Check sheet for the modelled part. Datum: model origin and axes. Units: mm. A direction names the side the tool comes from. Give positions to 0.01 mm unless a question says otherwise; leave off trailing zeros. Order: outer loops, then holes, each group sorted by start corner. A loop starts at its lowest first (then second) coordinate and runs counter-clockwise, first axis right, second up. Notation, with made-up numbers: (-17, -20) -> (30, -20) arc R30 cw to (30, 2) -> close; hole circle Ø2 at (62, 3). An arc over 180 degrees is marked (long way). Answer in a Markdown table with one row per item. Add a question column.
(1) Cross-section at D-D (x = 3.25). Record the cut outline in (y, z), then the cut area to 3 significant figures.
(2) Set-up check for faces 4 (the face through (1.5, 0, 1)), 5 (the face through (0, -2, 3)): record each of +Z, -Z, +X, -X, +Y, -Y from which the full face is reachable in a straight line by a thin tool's end or side.
(3) Go/stop test with a flat-tipped pin: pin 1 (1.5 mm diameter, centred on x = 3.5, z = 2, fed in from -Y). Record where the tip stops, or that it passes through.
(4) Cross-section at C-C (z = 0.7). Record the cut outline in (x, y), then the cut area to 3 significant figures.
(5) Cross-section at A-A (y = 0). Record the cut outline in (x, z), then the cut area to 3 significant figures.
(6) Release check for a two-part mould opening along X. For faces 1 (the face through (0, -2, 0)), 2 (the face through (-1.5, 0, 1)), 3 (the face through (-0.59, -4.46, 1.48)) record: released by +X, released by -X, zero draft, split by the parting line, or undercut.
(7) Thickness scan on L1, parallel to Y at x = -0.75, z = 1.6; L2, parallel to Y at x = 0.5, z = 0.65; L3, parallel to X at y = 1, z = 0.75. Record the ranges inside material, lowest first. Write a range as [from, to].
Autodesk Inventor part; units mm, degrees
ref_plane "YZ Plane" through (0, 0, 0) normal (1, 0, 0) x (0, 1, 0)
ref_plane "XZ Plane" through (0, 0, 0) normal (0, 1, 0) x (-1, 0, 0)
ref_plane "XY Plane" through (0, 0, 0) normal (0, 0, 1) x (1, 0, 0)
sketch "Esboço1" plane through (0, 0, 0) normal (0, 0, 1) x (1, 0, 0)
  circle A0 centre (0, 0) radius 4.5
  line L0 (-1.5, 1.5) -> (1.5, 1.5)
  line L1 (1.5, 1.5) -> (1.5, -1.5)
  line L2 (1.5, -1.5) -> (-1.5, -1.5)
  line L3 (-1.5, -1.5) -> (-1.5, 1.5)
extrude "Extrusão1" add sketch "Esboço1" along normal blind 3
properties part number "TRAVA_HELICE"
Answer below:
| question | item | result |
|---|---|---|
| 1 | outline | (-3.11, 0) -> (3.11, 0) -> (3.11, 3) -> (-3.11, 3) -> close |
| 1 | area | 18.7 mm² |
| 2 | face 4 | +Z, -Z |
| 2 | face 5 | +Z, +X, -X, +Y, -Y |
| 3 | pin 1 | stops at y = -3.56 |
| 4 | outline | circle Ø9 at (0, 0); hole (-1.5, -1.5) -> (1.5, -1.5) -> (1.5, 1.5) -> (-1.5, 1.5) -> close |
| 4 | area | 54.6 mm² |
| 5 | outline | (-4.5, 0) -> (-1.5, 0) -> (-1.5, 3) -> (-4.5, 3) -> close; (1.5, 0) -> (4.5, 0) -> (4.5, 3) -> (1.5, 3) -> close |
| 5 | area | 18.0 mm² |
| 6 | face 1 | zero draft |
| 6 | face 2 | undercut |
| 6 | face 3 | split by the parting line |
| 7 | L1 | y = [-4.44, -1.5], [1.5, 4.44] |
| 7 | L2 | y = [-4.47, -1.5], [1.5, 4.47] |
| 7 | L3 | x = [-4.39, -1.5], [1.5, 4.39] |
